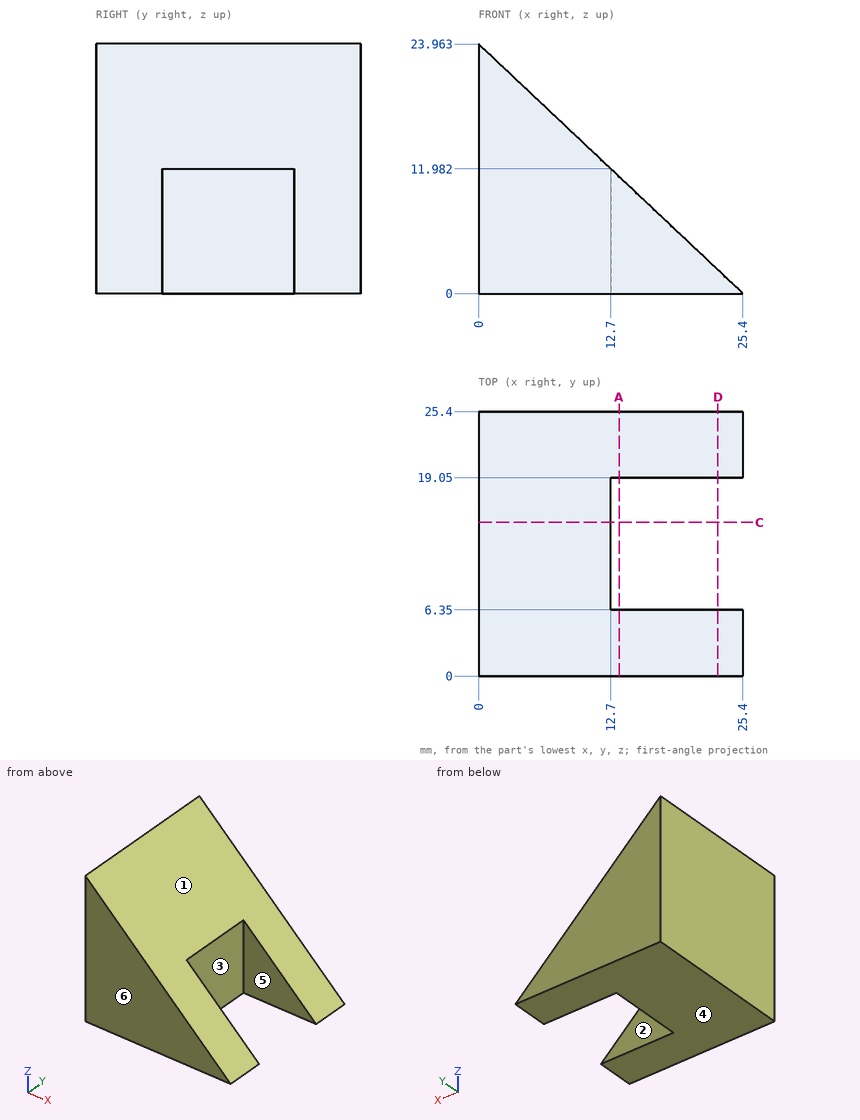
Can you work these out from the drawing? Everything is in mm from the part's minimum corner. A direction names the side the tool comes from. Coordinates: 2 decimals unless noted, no trailing zeros. Loops run counter-clockwise (first coordinate to the right, second up) from the corner with the lowest first, then second, coordinate; pieces in that order, holes last.
1) Which directions (+Z, -Z, +X, -X, +Y, -Y) give clear straight access to the entire face, cutting with the end or side of a thin tool? Please do the marked faces 1 and 2.
Reported:
face 1: +Z, +X, +Y, -Y
face 2: +Z, -Z, +X
2) Will these pins go through, and if not, where does the flat tip stop? pin 1 Ø6 at (x, y) = (11, 14.5) entering from +Z (1 decimal); pin 2 Ø5 at (y, z) = (21.5, 18.5) entering from +X; pin 3 Ø6 at (x, y) = (21, 3) entering from +Z.
Reported:
pin 1: stops at z = 16.4
pin 2: stops at x = 8.44
pin 3: stops at z = 6.98
3) Imagine slicing it at D-D (x = 23). List the corners of the cut face in (y, z) for me.
Reported:
outline: (0, 0) - (6.35, 0) - (6.35, 2.26) - (0, 2.26) - close; (19.05, 0) - (25.4, 0) - (25.4, 2.26) - (19.05, 2.26) - close
4) Please list where these lines run through material, in increasing order: line 1 along Y through (x, z) = (20.5, 4.25); line 2 along X through (y, z) = (9.5, 20); line 3 along X through (y, z) = (12.25, 7).
Reported:
line 1: y = 0 to 6.35, 19.05 to 25.4
line 2: x = 0 to 4.2
line 3: x = 0 to 12.7
5) Imagine slicing it at A-A (x = 13.5). List the corners of the cut face in (y, z) for me, and give its area (3 significant figures).
Reported:
outline: (0, 0) - (6.35, 0) - (6.35, 11.23) - (0, 11.23) - close; (19.05, 0) - (25.4, 0) - (25.4, 11.23) - (19.05, 11.23) - close
area: 143 mm2
6) Thinking about a two-plate mould opening in Y: for the marked faces 3, 4, 5 and 6, which applies, released by +Y, released by -Y, zero draft, split by the parting line, or undercut?
Reported:
face 3: undercut
face 4: zero draft
face 5: undercut
face 6: released by -Y
7) Imagine slicing it at C-C (y = 14.75). List the corners of the cut face in (x, z) for me.
Reported:
outline: (0, 0) - (12.7, 0) - (12.7, 11.98) - (0, 23.96) - close
